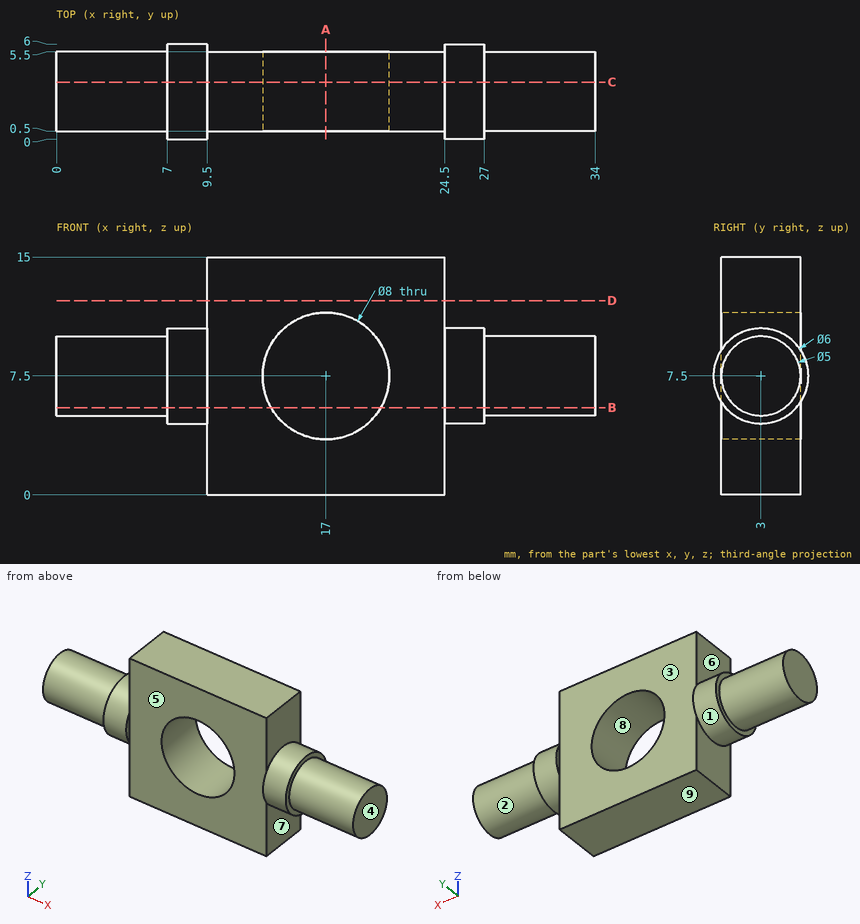
Verification items for this drawing (mm, ordinates from the low corner). A direction names the side the tool comes from. Coordinates: 2 decimals unless noted, no trailing zeros. Loops run counter-clockwise (first coordinate to the right, second up) from the corner with the lowest first, then second, coordinate; pieces in that order, holes last. Notation, with made-up numbers: (-10.5, 83) -> (25.5, 83) arc R4 ccw to (25.5, 87) -> close; hole circle Ø9 at (7.25, -26.75). An arc over 180 degrees is marked (long way). Put each result on its own line as item: value.
1. Section check A-A, the plane x = 17. Record the boundary of the cut face in (y, z), then the cut area to 3 significant figures.
Result set:
outline: (0.5, 0) -> (5.5, 0) -> (5.5, 3.5) -> (0.5, 3.5) -> close; (0.5, 11.5) -> (5.5, 11.5) -> (5.5, 15) -> (0.5, 15) -> close
area: 35.0 mm^2
2. Tool access check on the marked faces 1, 2, 3, 4 and 5. Record the directions out of +Z, -Z, +X, -X, +Y, -Y that give a thin tool (end or side, any length) a straight path to the whole face; none if there is none.
Result set:
face 1: -X
face 2: +X
face 3: +Z, -Z, +Y
face 4: +Z, -Z, +X, +Y, -Y
face 5: +Z, -Z, -Y
3. Gauge pin test, flat ends, axial feed: P1, Ø1.5, axis at y = 2.5, z = 10.5, coming from the +X side; P2, Ø2, axis at x = 22, z = 12.5, coming from the -Y side; P3, Ø1.5, axis at y = 3.5, z = 3.5, coming from the +X side; P4, Ø1, axis at y = 1, z = 2.5, coming from the -X side. Record the tip position at first contact, or that the pin passes through.
Result set:
P1: stops at x = 34
P2: stops at y = 0.5
P3: stops at x = 24.5
P4: stops at x = 9.5
4. Mould release check, pull along X, two halves, no side actions. Record for the marked faces 6, 7, 8 and 9: pulls with the +X half, pulls with the -X half, needs draft (parallel to the pull), parting line crosses it, or undercut.
Result set:
face 6: pulls with the -X half
face 7: pulls with the +X half
face 8: undercut
face 9: needs draft
5. Section check D-D, the plane z = 12.25. Record the boundary of the cut face in (x, y), then the cut area to 3 significant figures.
Result set:
outline: (9.5, 0.5) -> (24.5, 0.5) -> (24.5, 5.5) -> (9.5, 5.5) -> close
area: 75.0 mm^2
6. Thickness scan on line 1 (Z direction, x = 17, y = 4.15); line 2 (X direction, y = 3.15, z = 7.5); line 3 (Y direction, x = 14, z = 3.5). Record the ranges inside material, lowest first.
Result set:
line 1: z = 0 to 3.5, 11.5 to 15
line 2: x = 0 to 13, 21 to 34
line 3: y = 0.5 to 5.5
7. Section check C-C, the plane y = 3.6. Record the boundary of the cut face in (x, z), then the cut area to 3 significant figures.
Result set:
outline: (0, 5.07) -> (7, 5.07) -> (7, 4.56) -> (9.5, 4.56) -> (9.5, 0) -> (24.5, 0) -> (24.5, 4.56) -> (27, 4.56) -> (27, 5.07) -> (34, 5.07) -> (34, 9.93) -> (27, 9.93) -> (27, 10.44) -> (24.5, 10.44) -> (24.5, 15) -> (9.5, 15) -> (9.5, 10.44) -> (7, 10.44) -> (7, 9.93) -> (0, 9.93) -> close; hole circle Ø8 at (17, 7.5)
area: 272 mm^2
8. Section check B-B, the plane z = 5.5. Record the boundary of the cut face in (x, y), then the cut area to 3 significant figures.
Result set:
outline: (0, 1.5) -> (7, 1.5) -> (7, 0.76) -> (9.5, 0.76) -> (9.5, 0.5) -> (13.54, 0.5) -> (13.54, 5.5) -> (9.5, 5.5) -> (9.5, 5.24) -> (7, 5.24) -> (7, 4.5) -> (0, 4.5) -> close; (20.46, 0.5) -> (24.5, 0.5) -> (24.5, 0.76) -> (27, 0.76) -> (27, 1.5) -> (34, 1.5) -> (34, 4.5) -> (27, 4.5) -> (27, 5.24) -> (24.5, 5.24) -> (24.5, 5.5) -> (20.46, 5.5) -> close
area: 105 mm^2
